Build history of the part. All positions in model axes, mm. A direction names the side the tool comes from. Coordinates: 2 decimals unless noted, no trailing zeros. Loops run counter-clockwise (first coordinate to the right, second up) from the corner with the lowest first, then second, coordinate; pieces in that order, holes last.
(1) Two-plate mould, pull along X, no slides. Class faces 4 (the face through (-13.37, -1.36, 17.74)), 5 (the face through (-11, -1.6, 17)), 6 (the face through (-6, 0, 17)), 7 (the face through (-4.64, -9.37, 17.74)): pulls with the +X half, pulls with the -X half, needs draft (parallel to the pull), parting line crosses it, or undercut.
(2) Slice it at C-C (x = -11.25). Give the cut face in (y, z), and give its area (3 significant figures).
(3) Flat gauge pins, fed straight in: P1, Ø2, axis at x = -2, z = 10.5, coming from the -Y side; P2, Ø6, axis at x = -7.5, z = 16, coming from the +Y side; P3, Ø1.9, axis at y = -4.5, z = 21, coming from the +X side. Where does each tip first touch, or does it go through?
(4) Slice it at D-D (y = -3.25). Give the cut face in (x, z), and give its area (3 significant figures).
(5) Slice it at B-B (z = 4.5). Give the cut face in (x, y), and give its area (3 significant figures).
(6) Slice it at A-A (y = 8). Give the cut face in (x, z), and give its area (3 significant figures).
(7) Tool access for faces 1 (the face through (-12, 8, 17)), 2 (the face through (-7.6, -6, 17)), 3 (the face through (-1, -1.6, 17)): list every direction of +Z, -Z, +X, -X, +Y, -Y with a clear straight run to the whole face (end or side of a thin tool).
(8) Wall check: L1, parallel to X at y = 13.25, z = 28.5; L2, parallel to Y at x = -0.75, z = 8.5; L3, parallel to X at y = -7, z = 25.5. Give the ranges that are in metal, low to high.
from build123d import *

# Parameters (mm, degrees)
F0_W     = 3.2
F0_H     = 8
F1_DEPTH = 35
F2_R     = 0.8


# Not quite as in the source:
# - a feature names something its author has since deleted; it is built from what else it names


with BuildPart() as f1:
    # F0 (on Top) → F1 (new body)
    with BuildSketch(Plane.XY):
        Polygon((0, 16), (0, 0), (-12, 0), (-12, 16), (-13.6, 16), (-13.6, -1.6), (-7.6, -1.6), (-4.4, -1.6), (1.6, -1.6), (1.6, 16), align=None)
        with Locations((-6, -5.6)):
            Rectangle(F0_W, F0_H)
    extrude(amount=F1_DEPTH)

    # F2
    f2_edges = [f1.edges().sort_by_distance(p)[0] for p in [
        (1.6, -1.6, 17.5),
        (-13.6, -1.6, 17.5),
        (-7.6, -1.6, 17.5),
        (-4.4, -1.6, 17.5),
        (-7.6, -9.6, 17.5),
        (-4.4, -9.6, 17.5),
    ]]
    fillet(f2_edges, radius=F2_R)


solid = f1.part
Response values:
1. face 4: pulls with the -X half
1. face 5: needs draft
1. face 6: undercut
1. face 7: pulls with the +X half
2. outline: (-1.6, 0) - (0, 0) - (0, 35) - (-1.6, 35) - close
2. area: 56.0 mm2
3. P1: stops at y = -1.6
3. P2: stops at y = 0
3. P3: stops at x = -4.4
4. outline: (-7.6, 0) - (-4.4, 0) - (-4.4, 35) - (-7.6, 35) - close
4. area: 112 mm2
5. outline: (-13.6, -0.8) arc R0.8 ccw to (-12.8, -1.6) - (-8.4, -1.6) arc R0.8 cw to (-7.6, -2.4) - (-7.6, -8.8) arc R0.8 ccw to (-6.8, -9.6) - (-5.2, -9.6) arc R0.8 ccw to (-4.4, -8.8) - (-4.4, -2.4) arc R0.8 cw to (-3.6, -1.6) - (0.8, -1.6) arc R0.8 ccw to (1.6, -0.8) - (1.6, 16) - (0, 16) - (0, 0) - (-12, 0) - (-12, 16) - (-13.6, 16) - close
5. area: 101 mm2
6. outline: (-13.6, 0) - (-12, 0) - (-12, 35) - (-13.6, 35) - close; (0, 0) - (1.6, 0) - (1.6, 35) - (0, 35) - close
6. area: 112 mm2
7. face 1: +Z, -Z, +Y
7. face 2: +Z, -Z, -X, -Y
7. face 3: +Z, -Z, +X, -Y
8. L1: x = -13.6 to -12, 0 to 1.6
8. L2: y = -1.6 to 0
8. L3: x = -7.6 to -4.4
